from build123d import *

# Parameters (mm, degrees)
F0_R          = 6.096
F1_DEPTH      = 127
F2_R          = 2.921
F3_DEPTH      = 5.08
F3_DEPTH_BACK = 5.08
F4_R          = 2.54
F6_DEPTH      = 16.256
F7_R          = 1.27
F8_W          = 13.208
F8_H          = 15.24
F9_DEPTH      = 21.844


with BuildPart() as f1:
    # F0 (on Top) → F1 (new body)
    with BuildSketch(Plane.XY):
        with Locations((7.62, 0)):
            Circle(F0_R)
        with Locations((-7.62, 0)):
            Circle(F0_R)
    extrude(amount=F1_DEPTH)

    # F2 (on Right) → F3 (join, two sides)
    with BuildSketch(Plane.YZ) as f3_sk:
        with Locations((0, 111.602642)):
            Circle(F2_R)
    extrude(amount=F3_DEPTH)
    extrude(f3_sk.sketch, amount=-F3_DEPTH_BACK)

    # F4
    f4_edges = [f1.edges().sort_by_distance(p)[0] for p in [
        (-13.716, 0, 127),
        (1.524, 0, 127),
    ]]
    fillet(f4_edges, radius=F4_R)

    # F5 (on Top) → F6 (join)
    with BuildSketch(Plane.XY):
        with BuildLine():
            ThreePointArc((-15.875, -0.508), (-13.419969, -6.434969), (-7.493, -8.89))
            Line((-7.493, -8.89), (7.493, -8.89))
            ThreePointArc((7.493, -8.89), (13.419969, -6.434969), (15.875, -0.508))
            Line((15.875, -0.508), (15.875, 0.508))
            ThreePointArc((15.875, 0.508), (13.419969, 6.434969), (7.493, 8.89))
            Line((7.493, 8.89), (-7.493, 8.89))
            ThreePointArc((-7.493, 8.89), (-13.419969, 6.434969), (-15.875, 0.508))
            Line((-15.875, 0.508), (-15.875, -0.508))
        make_face()
    extrude(amount=-F6_DEPTH)

    # F7
    f7_edges = [f1.edges().sort_by_distance(p)[0] for p in [
        (0, -8.89, 0),
    ]]
    fillet(f7_edges, radius=F7_R)

    # F8 (on face) → F9 (join)
    with BuildSketch(Plane(origin=(0, 0, -16.256), x_dir=(1, 0, 0), z_dir=(0, 0, -1))):
        Rectangle(F8_W, F8_H)
    extrude(amount=F9_DEPTH)


solid = f1.part
Model file for the job. Use its own axes, mm. A direction names the side the tool comes from. Round coordinates to 2 decimals unless told otherwise and drop trailing zeros. Loops run counter-clockwise (first coordinate to the right, second up) from the corner with the lowest first, then second, coordinate; pieces in that order, holes last.
1. Wall check: probe 1 along Z at (x, y) = (1.5, 4.25); probe 2 along X at (y, z) = (-0.75, 116); probe 3 along X at (y, z) = (-2, 115). Give the ranges that are in metal, low to high.
Check values:
probe 1: z = -38.1 to 0
probe 2: x = -13.67 to -1.57, 1.57 to 13.67
probe 3: x = -13.38 to -1.86, 1.86 to 13.38
2. Band-saw the part on A-A, the plane z = 6. List the corners of the cut face in (x, y).
Check values:
outline: circle Ø12.19 at (-7.62, 0); circle Ø12.19 at (7.62, 0)
3. Tool access for faces 1 (the flat face through (0, 7.62, -27)), 2 (the cylindrical face through (-8.414, 6.044, 61.359)), 3 (the flat face through (6.604, 0, -27)), 4 (the flat face through (-6.604, 0, -27)): list every direction of +Z, -Z, +X, -X, +Y, -Y with a clear straight run to the whole face (end or side of a thin tool).
Check values:
face 1: -Z, +X, -X, +Y
face 2: none
face 3: -Z, +X, +Y, -Y
face 4: -Z, -X, +Y, -Y
4. Drop flat-ended pins along their axis: P1, Ø1.5, axis at y = -4, z = 79, coming from the +X side; P2, Ø8, axis at x = -6.5, z = 73.5, coming from the -Y side; P3, Ø10.5, axis at x = -1.5, z = -29, coming from the -Y side; P4, Ø10, axis at x = 10, y = -5.5, coming from the -Z side. Give the stop position or say it passes through.
Check values:
P1: stops at x = 12.78
P2: stops at y = -6.1
P3: stops at y = -7.62
P4: stops at z = -38.1
